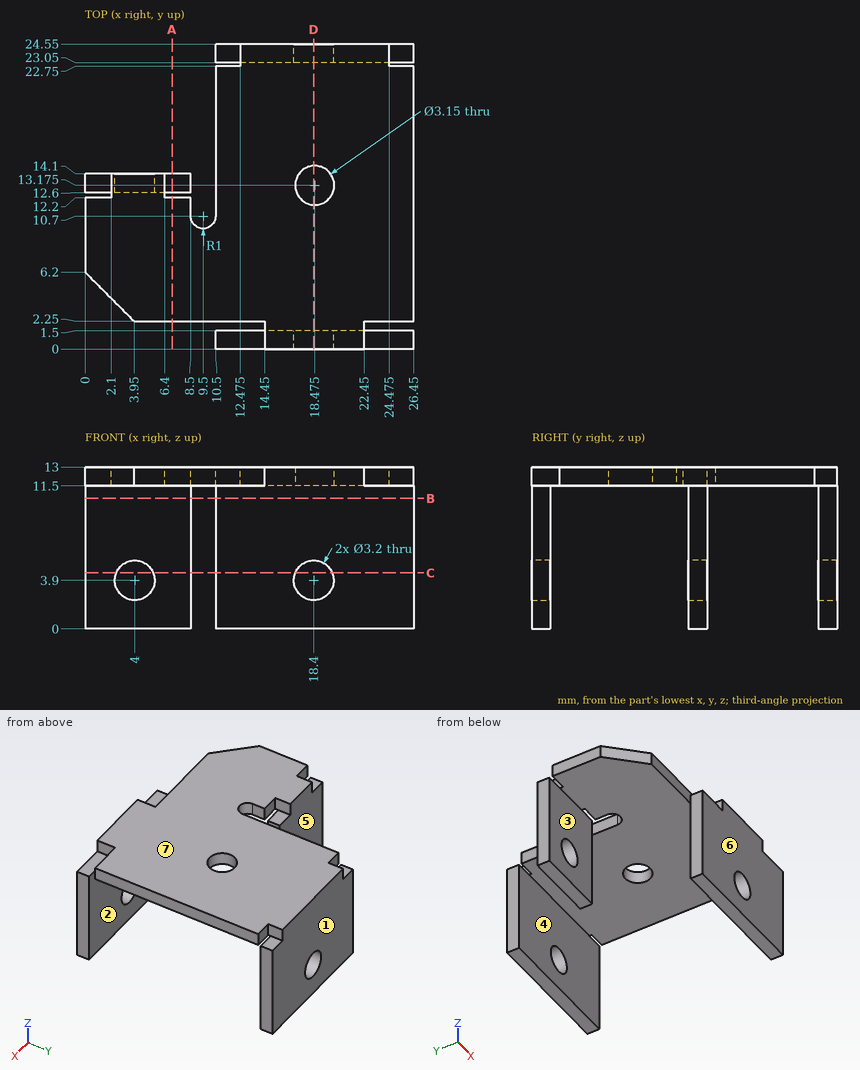
Here's the drawing with two shaded views (mm, measured from the low corner). I have some questions. A direction names the side the tool comes from. Coordinates: 2 decimals unless noted, no trailing zeros. Loops run counter-clockwise (first coordinate to the right, second up) from the corner with the lowest first, then second, coordinate; pieces in that order, holes last. Notation, with made-up numbers: (85.25, 15.25) -> (133.25, 15.25) arc R29 ccw to (133.25, 40.25) -> close; hole circle Ø11 at (-38, 72.5). An arc over 180 degrees is marked (long way). Use one line per item in the form item = value. Start each with the question number.
(1) If we section it at C-C (z = 4.5): Please give me the cut outline in (x, y).
(2) Will these pins go through, and if not, where does the flat tip stop? pin 1 (1.2 mm diameter, centred on x = 24, z = 12.5, fed in from -Y); pin 2 (1.6 mm diameter, centred on y = 23.5, z = 12.5, fed in from -X); pin 3 (4 mm diameter, centred on x = 3.5, z = 2, fed in from -Y); pin 4 (2.5 mm diameter, centred on x = 18.475, y = 13.175, fed in from -Z).
(3) If we section it at A-A (x = 7): Please give me the cut outline in (y, z).
(4) If we section it at D-D (x = 18.4): Please give me the cut outline in (y, z), then the cut area to 3 significant figures.
(5) Please list where these lines run through material, in increasing order: line 1 along Y through (x, z) = (17.5, 2); line 2 along X through (y, z) = (13.7, 3.9); line 3 along X through (y, z) = (0.6, 3.9).
(6) We'd pull the mould along Y, two halves only. Please class the marked faces 4, 5, 6 and 7: pulls with the +Y half, pulls with the -Y half, needs draft (parallel to the pull), parting line crosses it, or undercut.
(7) If we section it at B-B (z = 10.5): Please give me the cut outline in (x, y), then the cut area to 3 significant figures.
(8) On a 3-axis mill with a long thin cutter (end or side, diameter ignored), from which of +Z, -Z, +X, -X, +Y, -Y can I reach the whole of each face in a straight line? I mean the marked faces 1, 2 and 3. Say none if no direction works.
Verdict:
q1.outline = (0, 12.6) -> (2.52, 12.6) -> (2.52, 14.1) -> (0, 14.1) -> close; (5.48, 12.6) -> (8.5, 12.6) -> (8.5, 14.1) -> (5.48, 14.1) -> close; (10.5, 0) -> (16.92, 0) -> (16.92, 1.5) -> (10.5, 1.5) -> close; (10.5, 23.05) -> (16.92, 23.05) -> (16.92, 24.55) -> (10.5, 24.55) -> close; (19.88, 0) -> (26.45, 0) -> (26.45, 1.5) -> (19.88, 1.5) -> close; (19.88, 23.05) -> (26.45, 23.05) -> (26.45, 24.55) -> (19.88, 24.55) -> close
q2.pin_1 = 2.25
q2.pin_2 = 10.5
q2.pin_3 = 12.6
q2.pin_4 = through
q3.outline = (2.25, 11.5) -> (12.2, 11.5) -> (12.2, 13) -> (2.25, 13) -> close; (12.6, 0) -> (14.1, 0) -> (14.1, 11.5) -> (12.6, 11.5) -> close
q4.outline = (0, 0) -> (1.5, 0) -> (1.5, 2.3) -> (0, 2.3) -> close; (0, 5.5) -> (1.5, 5.5) -> (1.5, 11.5) -> (11.6, 11.5) -> (11.6, 13) -> (0, 13) -> close; (14.75, 11.5) -> (23.05, 11.5) -> (23.05, 5.5) -> (24.55, 5.5) -> (24.55, 13) -> (14.75, 13) -> close; (23.05, 0) -> (24.55, 0) -> (24.55, 2.3) -> (23.05, 2.3) -> close
q4.area = 57.0 mm²
q5.line_1 = 0 to 1.5, 23.05 to 24.55
q5.line_2 = 0 to 2.4, 5.6 to 8.5
q5.line_3 = 10.5 to 16.8, 20 to 26.45
q6.face_4 = undercut
q6.face_5 = pulls with the +Y half
q6.face_6 = pulls with the -Y half
q6.face_7 = needs draft
q7.outline = (0, 12.6) -> (8.5, 12.6) -> (8.5, 14.1) -> (0, 14.1) -> close; (10.5, 0) -> (26.45, 0) -> (26.45, 1.5) -> (10.5, 1.5) -> close; (10.5, 23.05) -> (26.45, 23.05) -> (26.45, 24.55) -> (10.5, 24.55) -> close
q7.area = 60.6 mm²
q8.face_1 = +Z, -Z, +X, -X, +Y
q8.face_2 = -Z, +X, -X
q8.face_3 = -Z, +X, -X, -Y
